For this review, use the dimensioned drawing (mm, ordinates from the lowest corner) and the shaded views. A direction names the side the tool comes from. Round coordinates to 2 decimals unless told otherwise and drop trailing zeros. Order: outer loops, then holes, each group sorted by start corner. A loop starts at its lowest first (then second) coordinate and runs counter-clockwise, first axis right, second up. Notation, with made-up numbers: (28.25, -14) -> (44.25, -14) arc R3 ccw to (44.25, -9) -> close; hole circle Ø2 at (63, 81). An arc over 180 degrees is marked (long way). Answer in a Markdown table with one row per item.
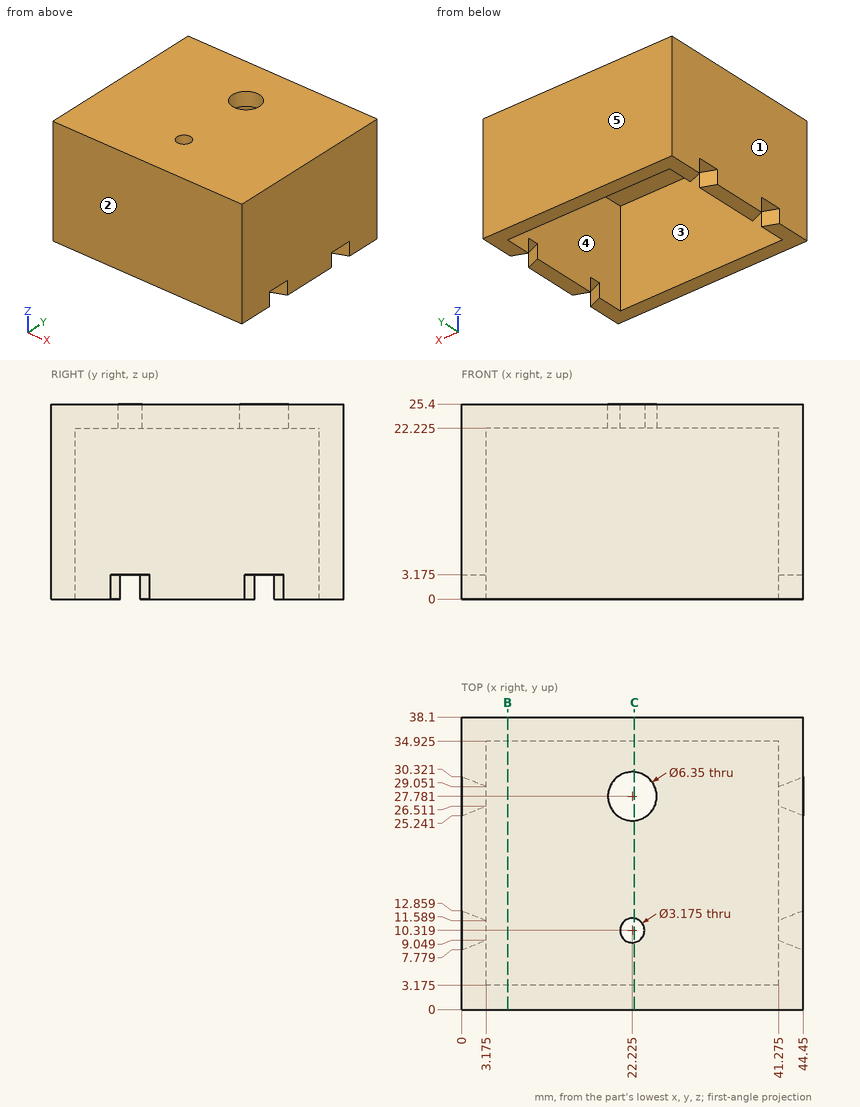
Q1. To check wall thickness, follow probe 1 along Y at (x, z) = (36, 3) (1 decimal); probe 2 along Z at (x, y) = (28.5, 21) (1 decimal); probe 3 along X at (y, z) = (26, 23.5). State the ranges of each line that lie inside material, in increasing order.
Answer key:
| item | result |
|---|---|
| probe 1 | y = 0 to 3.2, 34.9 to 38.1 |
| probe 2 | z = 22.2 to 25.4 |
| probe 3 | x = 0 to 19.6, 24.85 to 44.45 |
Q2. Clearance check with flat-ended pins moving along their axes: pin 1 Ø3 at (x, y) = (22.22, 10.32) entering from +Z; pin 2 Ø2 at (x, z) = (10.5, 9.5) entering from -Y; pin 3 Ø2.5 at (x, y) = (2, 28) entering from -Z (3 decimals). State where each tip first meets the part, or that it passes through.
Answer key:
| item | result |
|---|---|
| pin 1 | passes through |
| pin 2 | stops at y = 0 |
| pin 3 | stops at z = 3.175 |
Q3. Take a section at C-C, the plane x = 22.5. Write out the cut boundary in (y, z) (1 decimal), then the cut area to 3 significant figures.
Answer key:
| item | result |
|---|---|
| outline | (0, 0) -> (3.2, 0) -> (3.2, 22.2) -> (8.8, 22.2) -> (8.8, 25.4) -> (0, 25.4) -> close; (11.9, 22.2) -> (24.6, 22.2) -> (24.6, 25.4) -> (11.9, 25.4) -> close; (30.9, 22.2) -> (34.9, 22.2) -> (34.9, 0) -> (38.1, 0) -> (38.1, 25.4) -> (30.9, 25.4) -> close |
| area | 232 mm^2 |
Q4. The part is to be moulded in two halves that separate along Y. For the marked faces 1, 2 and 3, say which applies: +Y half, -Y half, draft (parallel to the pull), parting line (faces both ways), or undercut.
Answer key:
| item | result |
|---|---|
| face 1 | draft |
| face 2 | -Y half |
| face 3 | undercut |
Q5. Tool access review of the marked faces 4 and 5: name each direction out of +Z, -Z, +X, -X, +Y, -Y from which nothing blocks a thin tool from reaching the whole face with its end or side.
Answer key:
| item | result |
|---|---|
| face 4 | -Z |
| face 5 | +Z, -Z, +X, -X, +Y |
Q6. Take a section at B-B, the plane x = 6. Write out the cut boundary in (y, z) (1 decimal), then the cut area to 3 significant figures.
Answer key:
| item | result |
|---|---|
| outline | (0, 0) -> (3.2, 0) -> (3.2, 22.2) -> (34.9, 22.2) -> (34.9, 0) -> (38.1, 0) -> (38.1, 25.4) -> (0, 25.4) -> close |
| area | 262 mm^2 |
